```python
from build123d import *

# Parameters (mm, degrees)
ESQUISSE1_R        = 489.5
ESQUISSE1_R_2      = 443
ESQUISSE1_R_3      = 8.75
BOSS_EXTRU_1_DEPTH = 30


with BuildPart() as part:
    # Esquisse1 → Boss.-Extru.1 (new body)
    with BuildSketch(Plane.XY):
        Circle(ESQUISSE1_R)
        Circle(ESQUISSE1_R_2, mode=Mode.SUBTRACT)
        with Locations((-461, 0)):
            Circle(ESQUISSE1_R_3, mode=Mode.SUBTRACT)
        with Locations((-450.926043938, 95.847289467)):
            Circle(ESQUISSE1_R_3, mode=Mode.SUBTRACT)
        with Locations((-421.144455973, 187.505592458)):
            Circle(ESQUISSE1_R_3, mode=Mode.SUBTRACT)
        with Locations((-372.956834407, 270.969001307)):
            Circle(ESQUISSE1_R_3, mode=Mode.SUBTRACT)
        with Locations((-308.469209531, 342.589764545)):
            Circle(ESQUISSE1_R_3, mode=Mode.SUBTRACT)
        with Locations((-230.5, 399.237711145)):
            Circle(ESQUISSE1_R_3, mode=Mode.SUBTRACT)
        with Locations((-142.456834407, 438.437054012)):
            Circle(ESQUISSE1_R_3, mode=Mode.SUBTRACT)
        with Locations((-48.187621566, 458.474593765)):
            Circle(ESQUISSE1_R_3, mode=Mode.SUBTRACT)
        with Locations((48.187621566, 458.474593765)):
            Circle(ESQUISSE1_R_3, mode=Mode.SUBTRACT)
        with Locations((142.456834407, 438.437054012)):
            Circle(ESQUISSE1_R_3, mode=Mode.SUBTRACT)
        with Locations((230.5, 399.237711145)):
            Circle(ESQUISSE1_R_3, mode=Mode.SUBTRACT)
        with Locations((308.469209531, 342.589764545)):
            Circle(ESQUISSE1_R_3, mode=Mode.SUBTRACT)
        with Locations((372.956834407, 270.969001307)):
            Circle(ESQUISSE1_R_3, mode=Mode.SUBTRACT)
        with Locations((421.144455973, 187.505592458)):
            Circle(ESQUISSE1_R_3, mode=Mode.SUBTRACT)
        with Locations((450.926043938, 95.847289467)):
            Circle(ESQUISSE1_R_3, mode=Mode.SUBTRACT)
        with Locations((461, 0)):
            Circle(ESQUISSE1_R_3, mode=Mode.SUBTRACT)
        with Locations((450.926043938, -95.847289467)):
            Circle(ESQUISSE1_R_3, mode=Mode.SUBTRACT)
        with Locations((421.144455973, -187.505592458)):
            Circle(ESQUISSE1_R_3, mode=Mode.SUBTRACT)
        with Locations((372.956834407, -270.969001307)):
            Circle(ESQUISSE1_R_3, mode=Mode.SUBTRACT)
        with Locations((308.469209531, -342.589764545)):
            Circle(ESQUISSE1_R_3, mode=Mode.SUBTRACT)
        with Locations((230.5, -399.237711145)):
            Circle(ESQUISSE1_R_3, mode=Mode.SUBTRACT)
        with Locations((142.456834407, -438.437054012)):
            Circle(ESQUISSE1_R_3, mode=Mode.SUBTRACT)
        with Locations((48.187621566, -458.474593765)):
            Circle(ESQUISSE1_R_3, mode=Mode.SUBTRACT)
        with Locations((-48.187621566, -458.474593765)):
            Circle(ESQUISSE1_R_3, mode=Mode.SUBTRACT)
        with Locations((-142.456834407, -438.437054012)):
            Circle(ESQUISSE1_R_3, mode=Mode.SUBTRACT)
        with Locations((-230.5, -399.237711145)):
            Circle(ESQUISSE1_R_3, mode=Mode.SUBTRACT)
        with Locations((-308.469209531, -342.589764545)):
            Circle(ESQUISSE1_R_3, mode=Mode.SUBTRACT)
        with Locations((-372.956834407, -270.969001307)):
            Circle(ESQUISSE1_R_3, mode=Mode.SUBTRACT)
        with Locations((-421.144455973, -187.505592458)):
            Circle(ESQUISSE1_R_3, mode=Mode.SUBTRACT)
        with Locations((-450.926043938, -95.847289467)):
            Circle(ESQUISSE1_R_3, mode=Mode.SUBTRACT)
    extrude(amount=BOSS_EXTRU_1_DEPTH)


solid = part.part
```
CAD build for the part. Positions are in the model's coordinates, mm. Give positions to 0.01 mm unless a question says otherwise; leave off trailing zeros. Write each loop counter-clockwise with the first axis right and the second up, starting at its lowest first coordinate (ties: lowest second). Pieces come first, ordered by that corner, then holes. Notation, with made-up numbers: M 55,3 L 67,3 A19 ccw 67,17 Z; hole C 17,-4 d10. An arc over 180 degrees is marked long. Return JSON: item names as keys, results as strings. Group by question number.
(1) Flat gauge pins, fed straight in: pin 1 Ø12 at (x, z) = (-198.5, 3.5) entering from -Y; pin 2 Ø5 at (y, z) = (-192, 7) entering from +X; pin 3 Ø3 at (y, z) = (-182, 26.5) entering from +X. Where does each tip first touch, or does it go through?
(2) Drill centre lines: L1, parallel to X at y = 193, z = 19; L2, parallel to X at y = -264, z = 16.5; L3, parallel to X at y = -262, z = 11.75. Where is each one in solid material? Low to high. Write a range as [from, to].
(3) Band-saw the part on A-A (x = 0). Give the cut face in (y, z).
(4) Band-saw the part on B-B (y = -57.5). Give the cut face in (x, z), and give its area (3 significant figures).
(5) Band-saw the part on C-C (z = 6.5). State how many separate pieces and enclosed holes the cut face has, and give its area (3 significant figures).
Entries:
{
 "1": {"pin 1": "stops at y = -450.06", "pin 2": "stops at x = 451.33", "pin 3": "stops at x = 455.01"},
 "2": {"L1": "x = [-449.85, -427.95], [-414.33, -398.75], [398.75, 414.33], [427.95, 449.85]", "L2": "x = [-412.21, -378.25], [-367.67, -355.74], [355.74, 367.67], [378.25, 412.21]", "L3": "x = [-413.48, -357.22], [357.22, 413.48]"},
 "3": {"outline": "M -489.5,0 L -443,0 L -443,30 L -489.5,30 Z; M 443,0 L 489.5,0 L 489.5,30 L 443,30 Z"},
 "4": {"outline": "M -486.11,0 L -439.25,0 L -439.25,30 L -486.11,30 Z; M 439.25,0 L 486.11,0 L 486.11,30 L 439.25,30 Z", "area": "2,810 mm^2"},
 "5": {"separate pieces": "1", "enclosed holes": "31", "area": "129,000 mm^2"}
}
